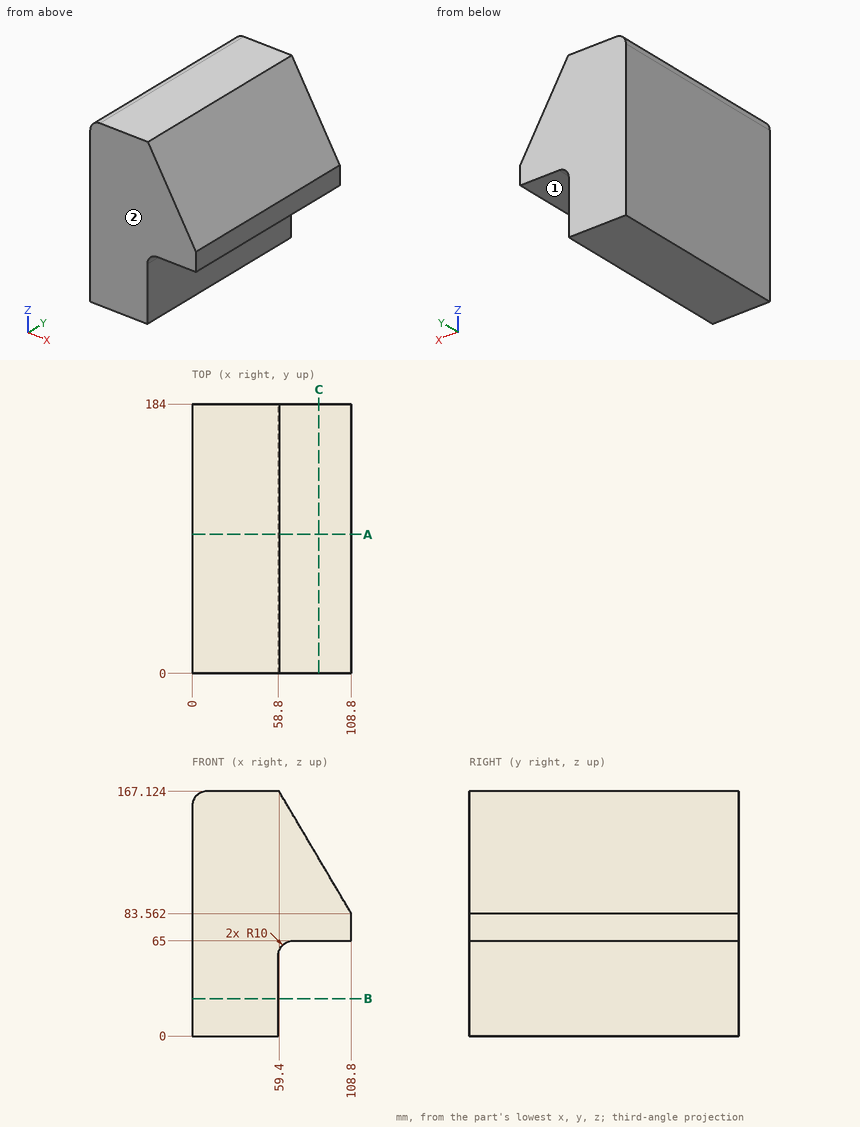
Here's the drawing with two shaded views (mm, measured from the low corner). I have some questions. A direction names the side the tool comes from. Round coordinates to 2 decimals unless told otherwise and drop trailing zeros. Loops run counter-clockwise (first coordinate to the right, second up) from the corner with the lowest first, then second, coordinate; pieces in that order, holes last. Notation, with made-up numbers: (15.25, -4) - (43.25, -4) arc R33 cw to (43.25, 24) - close; hole circle Ø7 at (15.5, -22.5). An arc over 180 degrees is marked (long way). Use CSV: the item, a comma, the result in double quotes. Start each with the question number.
1) For the marked faces 1 and 2, which set-ups out of +Z, -Z, +X, -X, +Y, -Y let a thin tool reach every point of the face, with its end or its side?
2) If we section it at A-A on y = 95: Write out the boundary of the cut face in (x, z), plus the area to 3 significant figures.
3) Please list where these lines run through material, in increasing order: probe 1 along X at (y, z) = (51, 38); probe 2 along X at (y, z) = (169, 158) (1 decimal); probe 3 along Z at (x, y) = (77.5, 155) (1 decimal). Write a range as [from, to].
4) If we section it at B-B on z = 25.5: Write out the boundary of the cut face in (x, y).
5) For pin 1 Ø1 at (y, z) = (46.5, 100) entering from +X, with a flat end and sliding along its axis, tell me the tip position at first contact or that it passes through.
6) If we section it at C-C on x = 86.5: Write out the boundary of the cut face in (y, z).
Geometry results:
1,face 1,"-Z, +X, +Y, -Y"
1,face 2,"+Z, -Z, +X, -X, -Y"
2,outline,"(0, 0) - (58.8, 0) - (58.8, 55) arc R10 cw to (68.8, 65) - (108.8, 65) - (108.8, 83.56) - (59.4, 167.12) - (10, 167.12) arc R10 ccw to (0, 157.12) - close"
2,area,"12,900 mm2"
3,probe 1,"x = [0, 58.8]"
3,probe 2,"x = [0, 64.8]"
3,probe 3,"z = [65, 136.5]"
4,outline,"(0, 0) - (58.8, 0) - (58.8, 184) - (0, 184) - close"
5,pin 1,"stops at x = 99.38"
6,outline,"(0, 65) - (184, 65) - (184, 121.28) - (0, 121.28) - close"
